Verification items for the finished model (mm, model axes). Face numbers are marked on the shaded views. A direction names the side the tool comes from. Give positions to 0.01 mm unless a question says otherwise; leave off trailing zeros. Write each loop counter-clockwise with the first axis right and the second up, starting at its lowest first coordinate (ties: lowest second). Pieces come first, ordered by that corner, then holes. Notation, with made-up numbers: (13, 20) - (61, 20) arc R13 cw to (61, 25) - close; hole circle Ø2 at (20, 0). An arc over 180 degrees is marked (long way). Answer as a JSON object with one key per item and string values. Group by question number.
Item 1: Scan lines: line 1 along Z through (x, y) = (-49, 41); line 2 along Y through (x, z) = (50.5, -56); line 3 along Y through (x, z) = (52, -104). Record each from-to range of solid material in increasing order. Write a range as [from, to].
Item 2: Draft check along Y on the marked faces 4, 5 and 6. Enter one of: +Y half, -Y half, draft (parallel to the pull), parting line (faces both ways), or undercut.
Item 3: Tool access check on the marked faces 1, 2 and 3. Record the directions out of +Z, -Z, +X, -X, +Y, -Y that give a thin tool (end or side, any length) a straight path to the whole face; none if there is none.
Item 4: Sectioned sample at B-B, the plane z = -296.5. Record the boundary of the cut face in (x, y), and give its area (3 significant figures).
Item 5: Sectioned sample at A-A, the plane y = -40. Record the boundary of the cut face in (x, z), and give its area (3 significant figures).
Item 6: Go/stop test with flat-tipped pins: pin 1 (12 mm diameter, centred on x = 111.5, z = -280.5, fed in from -Y); pin 2 (6 mm diameter, centred on x = -52, y = 51, fed in from +Z); pin 3 (4 mm diameter, centred on y = 69.5, z = -297, fed in from -X); pin 4 (8 mm diameter, centred on x = 36.5, z = -94, fed in from +Y). Record where each tip stops, or that it passes through.
Item 7: Sectioned sample at C-C, the plane y = -91. Record the boundary of the cut face in (x, z).
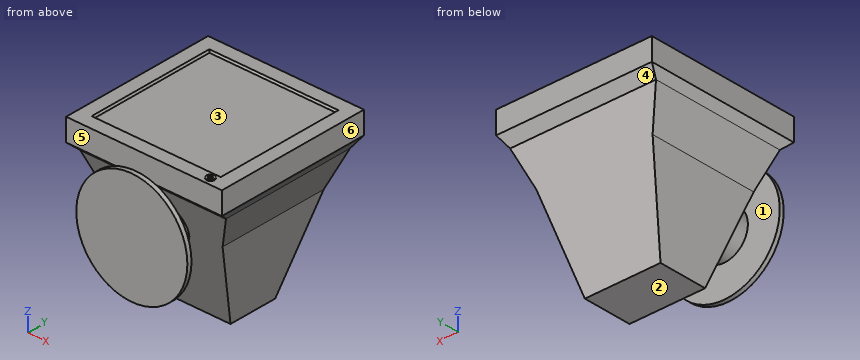
```python
from build123d import *

# Parameters (mm, degrees)
CROQUIS1_W                   = 350
CROQUIS1_H                   = 350
SALIENTE_EXTRUIR1_DEPTH      = 350
CROQUIS2_W                   = 290
CROQUIS2_H                   = 290
CORTAR_EXTRUIR1_DEPTH        = 5
CORTAR_EXTRUIR1_DRAFT        = -25
CORTAR_EXTRUIR2_REACH        = 527
CORTAR_EXTRUIR3_REACH        = 527
SALIENTE_EXTRUIR2_DEPTH      = 20
SALIENTE_EXTRUIR2_DEPTH_BACK = 85
CROQUIS5_R                   = 53.324987264
CROQUIS6_R                   = 125
SALIENTE_EXTRUIR3_DEPTH      = 10
SALIENTE_EXTRUIR3_TAPER      = 1
CROQUIS7_R                   = 9.05214815
SALIENTE_EXTRUIR4_DEPTH      = 2
CROQUIS8_R                   = 4.817972318
CORTAR_EXTRUIR4_DEPTH        = 2


with BuildPart() as part:
    # Croquis1 → Saliente-Extruir1 (new body)
    with BuildSketch(Plane.XY):
        Rectangle(CROQUIS1_W, CROQUIS1_H)
    extrude(amount=-SALIENTE_EXTRUIR1_DEPTH)


with BuildPart() as cortar_extruir1_tool:
    # Croquis2 → Cortar-Extruir1 (with draft: the straight prism first)
    with BuildSketch(Plane.XY):
        Rectangle(CROQUIS2_W, CROQUIS2_H)
    extrude(amount=-CORTAR_EXTRUIR1_DEPTH)
    # Cortar-Extruir1: the draft: its side faces are tilted about the plane it starts from
    cortar_extruir1_sides = [cortar_extruir1_tool.faces().sort_by_distance(p)[0] for p in [
        (-145, 0, -2.5),
        (0, -145, -2.5),
        (145, 0, -2.5),
        (0, 145, -2.5),
    ]]
    draft(cortar_extruir1_sides, Plane.XY, CORTAR_EXTRUIR1_DRAFT)


with BuildPart() as part_1:
    add(part.part)

    # Cortar-Extruir1: cut by cortar_extruir1_tool
    add(cortar_extruir1_tool.part, mode=Mode.SUBTRACT)

    # Croquis3 → Cortar-Extruir2 (cut, up to next)
    with BuildSketch(Plane(origin=(175, 0, 0), x_dir=(0, 0, -1), z_dir=(1, 0, 0)), mode=Mode.PRIVATE) as cortar_extruir2_sk1:
        Polygon((50, 175), (70, 152.639320225), (350, 55), (350, 175), align=None)
    cortar_extruir2_tool1 = extrude(cortar_extruir2_sk1.sketch, amount=-CORTAR_EXTRUIR2_REACH, mode=Mode.PRIVATE) & part_1.part
    # Croquis3 → Cortar-Extruir2 (cut, up to next)
    with BuildSketch(Plane(origin=(175, 0, 0), x_dir=(0, 0, -1), z_dir=(1, 0, 0)), mode=Mode.PRIVATE) as cortar_extruir2_sk2:
        Polygon((350, -175), (50, -175), (70, -152.639320225), (350, -55), align=None)
    cortar_extruir2_tool2 = extrude(cortar_extruir2_sk2.sketch, amount=-CORTAR_EXTRUIR2_REACH, mode=Mode.PRIVATE) & part_1.part
    add(cortar_extruir2_tool1.solids().sort_by_distance((175, 134.203352, -240.024387))[0], mode=Mode.SUBTRACT)
    add(cortar_extruir2_tool2.solids().sort_by_distance((175, -134.203352, -240.024387))[0], mode=Mode.SUBTRACT)

    # Croquis4 → Cortar-Extruir3 (cut, up to next)
    with BuildSketch(Plane(origin=(0, 175, 0), x_dir=(1, 0, 0), z_dir=(0, 1, 0)), mode=Mode.PRIVATE) as cortar_extruir3_sk1:
        Polygon((-85, 350), (-175, 350), (-175, 50), (-163.915974354, 70), (-130.682151375, 150.497096617), align=None)
    cortar_extruir3_tool1 = extrude(cortar_extruir3_sk1.sketch, amount=-CORTAR_EXTRUIR3_REACH, mode=Mode.PRIVATE) & part_1.part
    # Croquis4 → Cortar-Extruir3 (cut, up to next)
    with BuildSketch(Plane(origin=(0, 175, 0), x_dir=(1, 0, 0), z_dir=(0, 1, 0)), mode=Mode.PRIVATE) as cortar_extruir3_sk2:
        Polygon((130.682151375, 150.497096617), (85, 350), (175, 350), (175, 50), (163.915974354, 70), align=None)
    cortar_extruir3_tool2 = extrude(cortar_extruir3_sk2.sketch, amount=-CORTAR_EXTRUIR3_REACH, mode=Mode.PRIVATE) & part_1.part
    add(cortar_extruir3_tool1.solids().sort_by_distance((-143.088568, 175, -239.864683))[0], mode=Mode.SUBTRACT)
    add(cortar_extruir3_tool2.solids().sort_by_distance((143.088568, 175, -239.864683))[0], mode=Mode.SUBTRACT)

    # Croquis5 → Saliente-Extruir2 (add, two sides: drawn at the far end of the back side and taken through both)
    with BuildSketch(Plane.XZ.offset(175).offset(-SALIENTE_EXTRUIR2_DEPTH_BACK)):
        with Locations(Location((0, -150, 0), (0, 0, 270))):
            Circle(CROQUIS5_R)
    extrude(amount=SALIENTE_EXTRUIR2_DEPTH + SALIENTE_EXTRUIR2_DEPTH_BACK)

    # Croquis6 → Saliente-Extruir3 (add)
    with BuildSketch(Plane.XZ.offset(195)):
        with Locations((0, -150)):
            Circle(CROQUIS6_R)
    extrude(amount=SALIENTE_EXTRUIR3_DEPTH, taper=SALIENTE_EXTRUIR3_TAPER)

    # Croquis7 → Saliente-Extruir4 (add)
    with BuildSketch(Plane.XY):
        with Locations((134.907856816, -159.198773435)):
            Circle(CROQUIS7_R)
    extrude(amount=SALIENTE_EXTRUIR4_DEPTH)

    # Croquis8 → Cortar-Extruir4 (cut)
    with BuildSketch(Plane.XY.offset(2)):
        with Locations((134.907856816, -159.198773435)):
            Circle(CROQUIS8_R)
    extrude(amount=-CORTAR_EXTRUIR4_DEPTH, mode=Mode.SUBTRACT)


solid = part_1.part
```
Geometry check:
{
 "1": {"line 1": "[-350, -5]", "line 2": "[-205, -195], [-168.29, 168.29]", "line 3": "[-205, -195], [-140.78, 140.78]"},
 "2": {"face 4": "+Y half", "face 5": "undercut", "face 6": "draft"},
 "3": {"face 1": "none", "face 2": "-Z, +X, -X, +Y, -Y", "face 3": "+Z"},
 "4": {"outline": "(-97.25, -73.66) - (97.25, -73.66) - (97.25, 73.66) - (-97.25, 73.66) - close", "area": "28,700 mm^2"},
 "5": {"outline": "(-175, -50) - (-163.92, -70) - (-130.68, -150.5) - (-85, -350) - (85, -350) - (130.68, -150.5) - (163.92, -70) - (175, -50) - (175, 0) - (145, 0) - (142.67, -5) - (-142.67, -5) - (-145, 0) - (-175, 0) - close", "area": "89,600 mm^2"},
 "6": {"pin 1": "through", "pin 2": "z = -5", "pin 3": "x = -97.59", "pin 4": "y = 145.67"},
 "7": {"outline": "(-175, -50) - (-163.92, -70) - (-130.68, -150.5) - (-108.64, -246.76) - (108.64, -246.76) - (130.68, -150.5) - (163.92, -70) - (175, -50) - (175, 0) - (145, 0) - (142.67, -5) - (-142.67, -5) - (-145, 0) - (-175, 0) - close"}
}
